```python
from build123d import *

# Parameters (mm, degrees)
SKETCH_1_R      = 1.85
EXTRUDE_1_DEPTH = 3
CHAMFER_1_SIZE  = 0.1


with BuildPart() as part:
    # Эскиз1 → Бобышка-Вытянуть1 (new body)
    with BuildSketch(Plane(origin=(0, 0, 0), x_dir=(1, 0, 0), z_dir=(0, 1, 0))):
        Polygon((3.92598183, 0), (1.962990915, 3.4), (-1.962990915, 3.4), (-3.92598183, 0), (-1.962990915, -3.4), (1.962990915, -3.4), align=None)
        Circle(SKETCH_1_R, mode=Mode.SUBTRACT)
    extrude(amount=EXTRUDE_1_DEPTH)

    # Фаска1
    chamfer_1_edges = [part.edges().sort_by_distance(p)[0] for p in [
        (0, 3, -3.4),
        (-2.944486373, 3, -1.7),
        (-2.944486373, 3, 1.7),
        (-1.85, 0, 0),
        (-1.85, 3, 0),
        (0, 3, 3.4),
        (2.944486373, 3, 1.7),
        (0, 0, 3.4),
        (-2.944486373, 0, 1.7),
        (-2.944486373, 0, -1.7),
        (2.944486373, 3, -1.7),
        (0, 0, -3.4),
        (2.944486373, 0, -1.7),
        (2.944486373, 0, 1.7),
    ]]
    chamfer(chamfer_1_edges, length=CHAMFER_1_SIZE)


solid = part.part
```
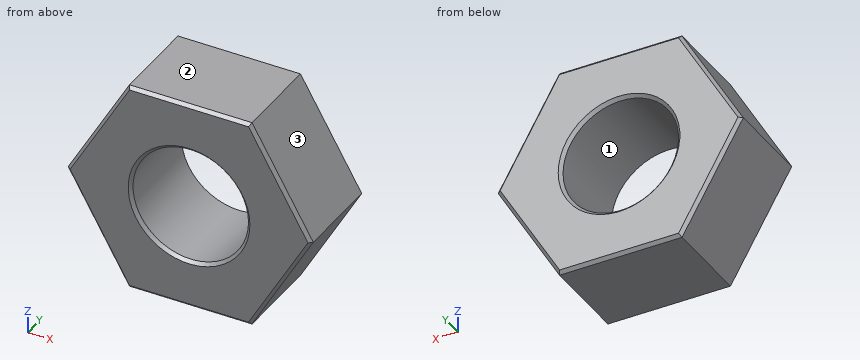
CAD build for the part. Positions are in the model's coordinates, mm. Face numbers are marked on the shaded views. Coordinates: 2 decimals unless noted, no trailing zeros. Write each loop counter-clockwise with the first axis right and the second up, starting at its lowest first coordinate (ties: lowest second). Pieces come first, ordered by that corner, then holes. Notation, with made-up numbers: (9.5, 35.25) -> (39.5, 35.25) arc R12 ccw to (39.5, 51.25) -> close; hole circle Ø5 at (87.5, 0.5). An arc over 180 degrees is marked (long way). Use CSV: the item, a comma, the result in double quotes. Start each with the question number.
Item 1: Wall check: probe 1 along Z at (x, y) = (0, 1.95); probe 2 along Z at (x, y) = (-1.5, 1.1); probe 3 along X at (y, z) = (0.65, -1.25). Give the ranges that are in metal, low to high.
Item 2: Band-saw the part on A-A, the plane x = 0. Write the cut outline in (y, z).
Item 3: Drop flat-ended pins along their axis: P1, Ø3.5, axis at x = 0, z = 0, coming from the -Y side; P2, Ø1, axis at y = 1.5, z = 2.5, coming from the +X side. Give the stop position or say it passes through.
Item 4: Band-saw the part on B-B, the plane y = 1.6. Write the cut outline in (x, z), plus the area to 3 significant figures.
Item 5: Band-saw the part on C-C, the plane z = 2.5. Write the cut outline in (x, y).
Item 6: Two-plate mould, pull along X, no slides. Class the marked faces 1, 2 and 3: +X half, -X half, draft (parallel to the pull), parting line (faces both ways), or undercut.
Response values:
1,probe 1,"z = -3.4 to -1.85, 1.85 to 3.4"
1,probe 2,"z = -3.4 to -1.08, 1.08 to 3.4"
1,probe 3,"x = -3.2 to -1.36, 1.36 to 3.2"
2,outline,"(0, -3.3) -> (0.1, -3.4) -> (2.9, -3.4) -> (3, -3.3) -> (3, -1.95) -> (2.9, -1.85) -> (0.1, -1.85) -> (0, -1.95) -> close; (0, 1.95) -> (0.1, 1.85) -> (2.9, 1.85) -> (3, 1.95) -> (3, 3.3) -> (2.9, 3.4) -> (0.1, 3.4) -> (0, 3.3) -> close"
3,P1,"passes through"
3,P2,"stops at x = 2.77"
4,outline,"(-3.93, 0) -> (-1.96, -3.4) -> (1.96, -3.4) -> (3.93, 0) -> (1.96, 3.4) -> (-1.96, 3.4) -> close; hole circle Ø3.7 at (0, 0)"
4,area,"29.3 mm2"
5,outline,"(-2.48, 0.1) -> (-2.37, 0) -> (2.37, 0) -> (2.48, 0.1) -> (2.48, 2.9) -> (2.37, 3) -> (-2.37, 3) -> (-2.48, 2.9) -> close"
6,face 1,"undercut"
6,face 2,"draft"
6,face 3,"+X half"
